Autodesk Fusion 360 part; units mm, degrees
sketch "Sketch1" plane through (0, 0, 0) normal (0, 0, 1) x (1, 0, 0)
  circle A0 centre (38.8472, 20.3675) radius 1.75
  circle A1 centre (38.8472, -0.0995) radius 1.525
  circle A2 centre (-37.6728, -20.3675) radius 1.75
  circle A3 centre (-37.6728, 20.3675) radius 1.75
  arc A4 (-38.6728, 24.3675) -> (-41.6728, 21.3675) centre (-38.6728, 21.3675) ccw
  line L0 (-38.6728, 24.3675) -> (39.8472, 24.3675)
  line L1 (-41.6728, -21.3675) -> (-41.6728, 21.3675)
  circle A5 centre (-37.6728, -0.0995) radius 1.525
  arc A6 (42.8472, 21.3675) -> (39.8472, 24.3675) centre (39.8472, 21.3675) ccw
  line L2 (42.8472, 21.3675) -> (42.8472, -21.3675)
  arc A7 (-41.6728, -21.3675) -> (-38.6728, -24.3675) centre (-38.6728, -21.3675) ccw
  line L3 (39.8472, -24.3675) -> (-38.6728, -24.3675)
  arc A8 (39.8472, -24.3675) -> (42.8472, -21.3675) centre (39.8472, -21.3675) ccw
  circle A9 centre (38.8472, -20.3675) radius 1.75
  line L4 (-20.9878, -3.6825) -> (-34.9878, -3.6825)
  line L5 (-34.9878, -3.6825) -> (-34.9878, -17.6825)
  line L6 (-34.9878, -17.6825) -> (-20.9878, -17.6825)
  line L7 (-20.9878, -17.6825) -> (-20.9878, -3.6825)
  line L8 (-1.9378, -17.6825) -> (-15.9378, -17.6825)
  line L9 (-15.9378, -17.6825) -> (-15.9378, -3.6825)
  line L10 (-15.9378, -3.6825) -> (-1.9378, -3.6825)
  line L11 (-1.9378, -3.6825) -> (-1.9378, -17.6825)
  line L12 (17.1122, -17.6825) -> (3.1122, -17.6825)
  line L13 (3.1122, -17.6825) -> (3.1122, -3.6825)
  line L14 (3.1122, -3.6825) -> (17.1122, -3.6825)
  line L15 (17.1122, -3.6825) -> (17.1122, -17.6825)
  line L16 (36.1622, -17.6825) -> (22.1622, -17.6825)
  line L17 (22.1622, -17.6825) -> (22.1622, -3.6825)
  line L18 (22.1622, -3.6825) -> (36.1622, -3.6825)
  line L19 (36.1622, -3.6825) -> (36.1622, -17.6825)
  line L20 (-21.4728, 2.8975) -> (-34.2728, 2.8975)
  line L21 (-34.2728, 2.8975) -> (-34.2728, 15.8975)
  line L22 (-34.2728, 15.8975) -> (-21.4728, 15.8975)
  line L23 (-21.4728, 15.8975) -> (-21.4728, 2.8975)
  line L24 (13.7272, 3.3125) -> (-9.2728, 3.3125)
  line L25 (-9.2728, 3.3125) -> (-9.2728, 15.4625)
  line L26 (-9.2728, 15.4625) -> (13.7272, 15.4625)
  line L27 (13.7272, 15.4625) -> (13.7272, 3.3125)
  point P0 (-27.9878, -10.6825)
  point P1 (-8.9378, -10.6825)
  point P2 (10.1122, -10.6825)
  point P3 (29.1622, -10.6825)
  point P4 (-27.8728, 9.3975)
  point P5 (2.2272, 9.3875)
  dimension "d44" = 3.05
  dimension "d45" = 3.05
  dimension "d46" = 20.268
  dimension "d47" = 3
  dimension "d48" = 3
  dimension "d49" = 3
  dimension "d50" = 3
  dimension "d51" = 3.5
  dimension "d52" = 4
  dimension "d53" = 1.4142
  dimension "d54" = 20.268
  dimension "d55" = 48.735
  dimension "d56" = 84.52
  dimension "d57" = 19.05
  dimension "d58" = 19.05
  dimension "d59" = 19.05
  dimension "d60" = 6.685
  dimension "d63" = 6.685
  dimension "d64" = 6.685
  dimension "d65" = 6.685
  dimension "d66" = 6.685
  dimension "d67" = 6.685
  dimension "d69" = 14
  dimension "d70" = 14
  dimension "d71" = 14
  dimension "d72" = 14
  dimension "d73" = 14
  dimension "d74" = 14
  dimension "d75" = 14
  dimension "d76" = 14
  dimension "d77" = 12.8
  dimension "d78" = 13
  dimension "d79" = 14.97
  dimension "d80" = 13.8
  dimension "d81" = 23
  dimension "d82" = 12.15
  dimension "d83" = 43.9
  dimension "d84" = 14.98
  dimension "d87" = 4
  dimension "d88" = 4
  dimension "d89" = 1.4142
  dimension "d92" = 4
  dimension "d93" = 1.4142
  dimension "d94" = 4
  dimension "d95" = 4
extrude "Extrude5" add sketch "Sketch1" along normal blind 2
extrude "Extrude1" [suppressed]
extrude "Extrude2" [suppressed]
extrude "Extrude3" [suppressed]
extrude "Extrude4" [suppressed]
equation "d53 = ( sqrt(2) ) * 1 mm"
equation "d89 = ( sqrt(2) ) * 1 mm"
Model file for the job. Use its own axes, mm. A direction names the side the tool comes from. Give positions to 0.01 mm unless a question says otherwise; leave off trailing zeros. Loops run counter-clockwise (first coordinate to the right, second up) from the corner with the lowest first, then second, coordinate; pieces in that order, holes last.
1) Saw through at B-B (x = -14). Write the cut outline in (y, z), plus the area to 3 significant figures.
2) Tool access for faces 1 (the flat face through (0, 0, 0)), 2 (the flat face through (-34.988, -11, 1)): list every direction of +Z, -Z, +X, -X, +Y, -Y with a clear straight run to the whole face (end or side of a thin tool).
3) Pull direction X, two halves, no side cores. Call faces 3 (the flat face through (17.112, -11, 1)), 4 (the cylindrical face through (41.992, -23.465, 0.986)), 5 (the flat face through (0, 24.368, 1)): +X half, -X half, draft (parallel to the pull), parting line (faces both ways), or undercut.
4) Saw through at A-A (y = -14.5). Write the cut outline in (x, z).
5) Flat gauge pin, fed straight in: pin 1 Ø1.5 at (x, y) = (16.5, -18) entering from -Z. Where does the tip first touch, or does it go through?
6) Saw through at C-C (x = 7). Write the cut outline in (y, z), plus the area to 3 significant figures.
7) Saw through at D-D (y = 9). Write the cut outline in (x, z).
8) Wall check: line 1 (Y direction, x = -6.5, z = 1.7); line 2 (X direction, y = 20.5, z = 1.85); line 3 (X direction, y = -5, z = 0.3). Give the ranges that are in metal, low to high.
Answer block:
1. outline: (-24.37, 0) - (-17.68, 0) - (-17.68, 2) - (-24.37, 2) - close; (-3.68, 0) - (24.37, 0) - (24.37, 2) - (-3.68, 2) - close
1. area: 69.5 mm2
2. face 1: -Z, +X, -X, +Y, -Y
2. face 2: +Z, -Z
3. face 3: undercut
3. face 4: +X half
3. face 5: draft
4. outline: (-41.67, 0) - (-34.99, 0) - (-34.99, 2) - (-41.67, 2) - close; (-20.99, 0) - (-15.94, 0) - (-15.94, 2) - (-20.99, 2) - close; (-1.94, 0) - (3.11, 0) - (3.11, 2) - (-1.94, 2) - close; (17.11, 0) - (22.16, 0) - (22.16, 2) - (17.11, 2) - close; (36.16, 0) - (42.85, 0) - (42.85, 2) - (36.16, 2) - close
5. pin 1: stops at z = 0
6. outline: (-24.37, 0) - (-17.68, 0) - (-17.68, 2) - (-24.37, 2) - close; (-3.68, 0) - (3.31, 0) - (3.31, 2) - (-3.68, 2) - close; (15.46, 0) - (24.37, 0) - (24.37, 2) - (15.46, 2) - close
6. area: 45.2 mm2
7. outline: (-41.67, 0) - (-34.27, 0) - (-34.27, 2) - (-41.67, 2) - close; (-21.47, 0) - (-9.27, 0) - (-9.27, 2) - (-21.47, 2) - close; (13.73, 0) - (42.85, 0) - (42.85, 2) - (13.73, 2) - close
8. line 1: y = -24.37 to -17.68, -3.68 to 3.31, 15.46 to 24.37
8. line 2: x = -41.67 to -39.42, -35.93 to 37.1, 40.59 to 42.85
8. line 3: x = -41.67 to -34.99, -20.99 to -15.94, -1.94 to 3.11, 17.11 to 22.16, 36.16 to 42.85
